Design review of the part built by this model. Coordinates are the model's own, in mm. Face numbers are marked on the shaded views. A direction names the side the tool comes from. Coordinates: 2 decimals unless noted, no trailing zeros. Write each loop counter-clockwise with the first axis right and the second up, starting at its lowest first coordinate (ties: lowest second). Pieces come first, ordered by that corner, then holes. Notation, with made-up numbers: (0.25, -32) - (20.25, -32) arc R28 cw to (20.25, -3) - close; hole circle Ø11 at (6.25, -28.75). An arc over 180 degrees is marked (long way). One line per item, written item: value.
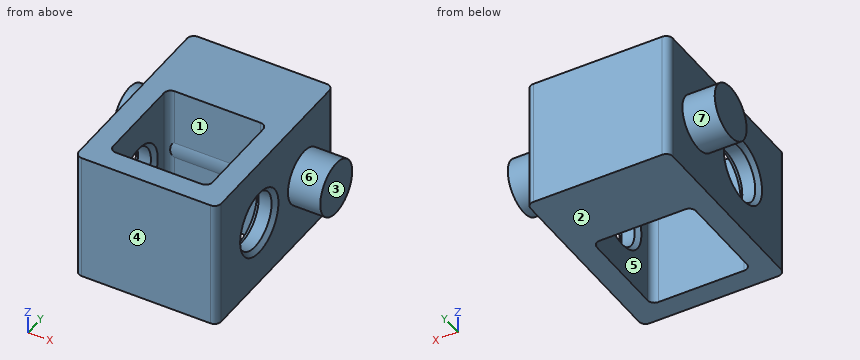
from build123d import *

# Parameters (mm, degrees)
SKETCH1_W                = 66
SKETCH1_H                = 66
BOSS_EXTRUDE1_DEPTH      = 60
SHELL1_T                 = -10
FILLET2_R                = 3.1
SKETCH2_W                = 60
SKETCH2_H                = 25
BOSS_EXTRUDE2_DEPTH      = 66
FILLET3_R                = 3.1
BOSS_EXTRUDE4_DEPTH      = 48
BOSS_EXTRUDE4_DEPTH_BACK = 48
SKETCH3_R                = 12.5
CUT_EXTRUDE1_DEPTH       = 110.567330952
CUT_EXTRUDE1_DEPTH_BACK  = 110.567330952
SKETCH4_R                = 13
CHAMFER1_SIZE            = 2


with BuildPart() as part:
    # Sketch1 → Boss-Extrude1 (new body)
    with BuildSketch(Plane.XY):
        Rectangle(SKETCH1_W, SKETCH1_H)
    extrude(amount=BOSS_EXTRUDE1_DEPTH)

    # Shell1
    shell1_openings = [part.faces().sort_by_distance(p)[0] for p in [
        (0, 0, 60),
        (0, 0, 0),
    ]]
    offset(amount=SHELL1_T, openings=shell1_openings, kind=Kind.INTERSECTION)

    # Fillet2
    fillet2_edges = [part.edges().sort_by_distance(p)[0] for p in [
        (23, -23, 30),
        (23, 23, 30),
        (-23, 23, 30),
        (-23, -23, 30),
    ]]
    fillet(fillet2_edges, radius=FILLET2_R)

    # Sketch2 → Boss-Extrude2 (add)
    with BuildSketch(Plane(origin=(33, 0, 0), x_dir=(0, 0, -1), z_dir=(1, 0, 0))):
        with Locations((-30, 45.5)):
            Rectangle(SKETCH2_W, SKETCH2_H)
    extrude(amount=-BOSS_EXTRUDE2_DEPTH)

    # Fillet3
    fillet3_edges = [part.edges().sort_by_distance(p)[0] for p in [
        (33, 58, 30),
        (-33, 58, 30),
        (33, -33, 30),
        (-33, -33, 30),
    ]]
    fillet(fillet3_edges, radius=FILLET3_R)

    # Sketch3 → Boss-Extrude4 (add, two sides: drawn at the far end of the back side and taken through both)
    with BuildSketch(Plane(origin=(0, 0, 0), x_dir=(0, 0, -1), z_dir=(1, 0, 0)).offset(-BOSS_EXTRUDE4_DEPTH_BACK)):
        with Locations((-30, 34.952906867)):
            Circle(SKETCH3_R)
    extrude(amount=BOSS_EXTRUDE4_DEPTH + BOSS_EXTRUDE4_DEPTH_BACK)

    # Sketch4 → Cut-Extrude1 (cut, two sides: drawn at the far end of the back side and taken through both)
    with BuildSketch(Plane.ZY.offset(-23).offset(-CUT_EXTRUDE1_DEPTH_BACK)):
        with Locations(Location((30, 0, 0), (0, 0, 180))):
            Circle(SKETCH4_R)
    extrude(amount=CUT_EXTRUDE1_DEPTH + CUT_EXTRUDE1_DEPTH_BACK, mode=Mode.SUBTRACT)

    # Chamfer1
    chamfer1_edges = [part.edges().sort_by_distance(p)[0] for p in [
        (33, 0, 43),
        (-33, 0, 43),
        (-23, 0, 43),
        (23, 0, 43),
    ]]
    chamfer(chamfer1_edges, length=CHAMFER1_SIZE)


solid = part.part
1. Insertion check: pin 1 Ø12 at (y, z) = (-4.5, 19.5) entering from -X; pin 2 Ø1.5 at (y, z) = (-1, 15.5) entering from +X; pin 3 Ø4 at (y, z) = (-4, 42) entering from -X. Each pin has a flat end and moves straight along its axis. Give the tip position at first contact, or say it passes through.
Answer block:
pin 1: stops at x = -33
pin 2: stops at x = 33
pin 3: stops at x = -32.65
2. Consider section C-C, the plane x = 28.5. Write out the cut boundary in (y, z).
Answer block:
outline: (-33, 0) - (58, 0) - (58, 60) - (-33, 60) - close; hole circle Ø26 at (0, 30)
3. Consider section B-B, the plane z = 13. Write out the cut boundary in (x, y), then the cut area to 3 significant figures.
Answer block:
outline: (-33, -29.9) arc R3.1 ccw to (-29.9, -33) - (29.9, -33) arc R3.1 ccw to (33, -29.9) - (33, 54.9) arc R3.1 ccw to (29.9, 58) - (-29.9, 58) arc R3.1 ccw to (-33, 54.9) - close; hole (-23, -19.9) arc R3.1 ccw to (-19.9, -23) - (19.9, -23) arc R3.1 ccw to (23, -19.9) - (23, 19.9) arc R3.1 ccw to (19.9, 23) - (-19.9, 23) arc R3.1 ccw to (-23, 19.9) - close
area: 3,890 mm^2
4. Consider section D-D, the plane y = 33. Write out the cut boundary in (x, z).
Answer block:
outline: (-48, 17.65) - (-33, 17.65) - (-33, 0) - (33, 0) - (33, 17.65) - (48, 17.65) - (48, 42.35) - (33, 42.35) - (33, 60) - (-33, 60) - (-33, 42.35) - (-48, 42.35) - close
5. For the marked faces 4, 5, 6 and 7, list the 3-axis set-ups (+Z, -Z, +X, -X, +Y, -Y) from which the entire face can be reached by the end or side of a thin tool; tool diameter is ignored.
Answer block:
face 4: +Z, -Z, +X, -X, -Y
face 5: +Z, -Z
face 6: +X
face 7: -X
6. Consider section A-A, the plane y = 0. Write out the cut boundary in (x, z).
Answer block:
outline: (-33, 0) - (-23, 0) - (-23, 15) - (-25, 17) - (-31, 17) - (-33, 15) - close; (-33, 45) - (-31, 43) - (-25, 43) - (-23, 45) - (-23, 60) - (-33, 60) - close; (23, 0) - (33, 0) - (33, 15) - (31, 17) - (25, 17) - (23, 15) - close; (23, 45) - (25, 43) - (31, 43) - (33, 45) - (33, 60) - (23, 60) - close
7. Wall thickness on line 1 along Y through (x, z) = (28, 30); line 2 along Y through (x, z) = (8, 35); line 3 along X through (y, z) = (-6.5, 5.5): over which ranges is each line inside the solid? List them lowest first.
Answer block:
line 1: y = -33 to -13, 13 to 58
line 2: y = -33 to -23, 23 to 58
line 3: x = -33 to -23, 23 to 33
8. Mouldability with a two-part tool opening along X and no side actions: class the marked faces 1, 2 and 3 as released by +X, released by -X, zero draft, split by the parting line, or undercut.
Answer block:
face 1: undercut
face 2: zero draft
face 3: released by +X
